Geometry: final body of the model. Coordinates: model frame, mm. Face numbers are marked on the shaded views. A direction names the side the tool comes from. Give positions to 0.01 mm unless a question says otherwise; leave off trailing zeros. Write each loop counter-clockwise with the first axis right and the second up, starting at its lowest first coordinate (ties: lowest second). Pieces come first, ordered by that corner, then holes. Notation, with made-up numbers: M 86,-26 L 131,-26 A17 cw 131,1 Z; hole C 58,-9.5 d5. An arc over 180 degrees is marked long. Use a Markdown table: item, result. Add a question column.
(1) Cut plane C-C (y = -9). Output: boundary loops of the cut face in (x, z).
(2) Material intervals for L1, parallel to Z at x = -4, y = -12; L2, parallel to X at y = -38, z = 2; L3, parallel to Y at x = 23.5, z = 10.5, sorted ascending.
(3) Reachability of the marked faces 1, 2 and 3 from +Z, -Z, +X, -X, +Y, -Y: full face, straight path, thin tool, end or side. Return the list, or none.
(4) Pin query (flat end, axial travel): pin 1 Ø19.5 at (x, z) = (-9.5, 25) entering from -Y; pin 2 Ø1 at (x, y) = (19.5, -45.5) entering from +Z; pin 3 Ø6 at (x, y) = (19.5, -46.5) entering from +Z. Return the tip coordinate at first contact, or that it passes through.
(5) Draft query along X for the marked faces 4, 5 and 6. Return one class per face: released by +X, released by -X, zero draft, split by the parting line, or undercut.
(6) Cut plane A-A (y = -47). Output: boundary loops of the cut face in (x, z).
(7) Cut plane D-D (x = -36). Output: boundary loops of the cut face in (y, z).
(8) Cut plane B-B (z = 25). Output: boundary loops of the cut face in (x, y), plus the area to 3 significant figures.
```python
from build123d import *

# Parameters (mm, degrees)
F0_W     = 30
F0_H     = 40
F1_DEPTH = 20
F3_DEPTH = 40


with BuildPart() as f1:
    # F0 (on Front) → F1 (new body)
    with BuildSketch(Plane.XZ):
        Rectangle(F0_W, F0_H)
        Polygon((15, 45), (15, 20), (15, -20), (45, -20), (45, 45), align=None)
        Polygon((-15, -20), (-15, 20), (-15, 45), (-45, 45), (-45, -20), align=None)
    extrude(amount=F1_DEPTH)

    # F2 (on face) → F3 (join)
    with BuildSketch(Plane.XZ.offset(20)):
        Polygon((-15, -20), (-45, 45), (-45, -20), align=None)
        Polygon((45, 45), (15, -20), (45, -20), align=None)
    extrude(amount=F3_DEPTH)


solid = f1.part
```
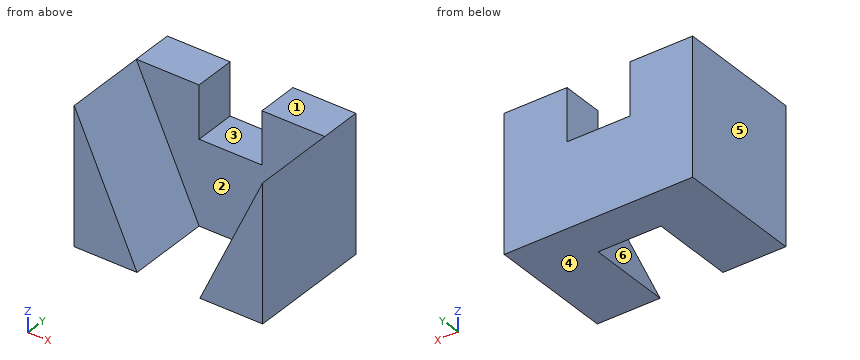
Answer list:
| question | item | result |
|---|---|---|
| 1 | outline | M -45,-20 L 45,-20 L 45,45 L 15,45 L 15,20 L -15,20 L -15,45 L -45,45 Z |
| 2 | L1 | -20 to 20 |
| 2 | L2 | -45 to -25.15, 25.15 to 45 |
| 2 | L3 | -20 to 0 |
| 3 | face 1 | +Z, +X, -X, +Y, -Y |
| 3 | face 2 | +Z, -Y |
| 3 | face 3 | +Z, +Y, -Y |
| 4 | pin 1 | y = -20 |
| 4 | pin 2 | z = -9.17 |
| 4 | pin 3 | z = -3.75 |
| 5 | face 4 | zero draft |
| 5 | face 5 | released by -X |
| 5 | face 6 | undercut |
| 6 | outline | M -45,-20 L -15,-20 L -45,45 Z; M 15,-20 L 45,-20 L 45,45 Z |
| 7 | outline | M -60,-20 L 0,-20 L 0,45 L -20,45 L -20,25.5 L -60,25.5 Z |
| 8 | outline | M -45,-60 L -35.77,-60 L -35.77,-20 L -15,-20 L -15,0 L -45,0 Z; M 15,-20 L 35.77,-20 L 35.77,-60 L 45,-60 L 45,0 L 15,0 Z |
| 8 | area | 1,940 mm² |
